from build123d import *

# Parameters (mm, degrees)
BOSS_EXTRUDE1_DEPTH = 20
SKETCH3_R           = 1
CUT_EXTRUDE1_DEPTH  = 10
SKETCH4_R           = 1
CUT_EXTRUDE2_DEPTH  = 10


with BuildPart() as part:
    # Sketch1 → Boss-Extrude1 (new body)
    with BuildSketch(Plane.XY):
        Polygon((0, 0), (58, 0), (58, 60), (61, 60), (61, -3), (-3, -3), (-3, 60), (0, 60), align=None)
    extrude(amount=-BOSS_EXTRUDE1_DEPTH)

    # Sketch3 → Cut-Extrude1 (cut)
    with BuildSketch(Plane(origin=(61, 0, 0), x_dir=(0, 0, -1), z_dir=(1, 0, 0))):
        with Locations((10, 57.541077174)):
            Circle(SKETCH3_R)
        with Locations((10, 30.375)):
            Circle(SKETCH3_R)
        Polygon((10, 32.55), (16, 32.55), (16, 55.366077174), (10, 55.366077174), (4, 55.366077174), (4, 32.55), align=None)
    extrude(amount=-CUT_EXTRUDE1_DEPTH, mode=Mode.SUBTRACT)

    # Sketch4 → Cut-Extrude2 (cut)
    with BuildSketch(Plane(origin=(0, 0, 0), x_dir=(1, 0, 0), z_dir=(0, 1, 0))):
        with Locations((19, 10)):
            Circle(SKETCH4_R)
        with Locations((39, 10)):
            Circle(SKETCH4_R)
    extrude(amount=-CUT_EXTRUDE2_DEPTH, mode=Mode.SUBTRACT)


solid = part.part
Check sheet for the modelled part. Datum: model origin and axes. Units: mm. A direction names the side the tool comes from. Give positions to 0.01 mm unless a question says otherwise; leave off trailing zeros. Order: outer loops, then holes, each group sorted by start corner. A loop starts at its lowest first (then second) coordinate and runs counter-clockwise, first axis right, second up. Notation, with made-up numbers: (-24, 47) - (27, 47) arc R11 ccw to (27, 66) - close; hole circle Ø9 at (-30.75, 23). An arc over 180 degrees is marked (long way). Answer as CSV lines item,"result".
1. Go/stop test with flat-tipped pins: P1, Ø3, axis at y = 57.54, z = -10, coming from the +X side; P2, Ø2.5, axis at x = 19, z = -10, coming from the +Y side. Record where each tip stops, or that it passes through.
Result sheet:
P1,"x = 61"
P2,"y = 0"
2. Section check D-D (y = 42.5). Record the boundary of the cut face in (x, z), then the cut area to 3 significant figures.
Result sheet:
outline,"(-3, -20) - (0, -20) - (0, 0) - (-3, 0) - close; (58, -20) - (61, -20) - (61, -16) - (58, -16) - close; (58, -4) - (61, -4) - (61, 0) - (58, 0) - close"
area,"84.0 mm²"
3. Mould release check, pull along Y, two halves, no side actions. Record for faces 1 (the face through (59, 60, -10)), 2 (the face through (60, 32.55, -10)), 3 (the face through (18.263, -1.479, -10.676)), 4 (the face through (60, 44, -16)): released by +Y, released by -Y, zero draft, split by the parting line, or undercut.
Result sheet:
face 1,"released by +Y"
face 2,"undercut"
face 3,"zero draft"
face 4,"undercut"
4. Tool access check on faces 5 (the face through (59.521, 31.366, -9.87)), 6 (the face through (29, -2, 0)), 7 (the face through (29, 0, -10)). Record the directions out of +Z, -Z, +X, -X, +Y, -Y that give a thin tool (end or side, any length) a straight path to the whole face; none if there is none.
Result sheet:
face 5,"+X"
face 6,"+Z, +X, -X, +Y, -Y"
face 7,"+Z, -Z, +Y"
5. Section check A-A (x = 19). Record the boundary of the cut face in (y, z).
Result sheet:
outline,"(-3, -20) - (0, -20) - (0, -11) - (-3, -11) - close; (-3, -9) - (0, -9) - (0, 0) - (-3, 0) - close"
6. Scan lines: probe 1 along X at (y, z) = (-1.4, -10); probe 2 along Y at (x, z) = (60.2, -10) (3 decimals); probe 3 along X at (y, z) = (17.5, -10.75). Record each from-to range of solid material in increasing order. Write a range as from..to.
Result sheet:
probe 1,"-3..18, 20..38, 40..61"
probe 2,"-3..29.375, 31.375..32.55, 55.366..56.541, 58.541..60"
probe 3,"-3..0, 58..61"
7. Section check C-C (y = 17.5). Record the boundary of the cut face in (x, z), then the cut area to 3 significant figures.
Result sheet:
outline,"(-3, -20) - (0, -20) - (0, 0) - (-3, 0) - close; (58, -20) - (61, -20) - (61, 0) - (58, 0) - close"
area,"120 mm²"
8. Section check B-B (z = -10). Record the boundary of the cut face in (x, y) (3 decimals), then the cut area to 3 significant figures.
Result sheet:
outline,"(-3, -3) - (18, -3) - (18, 0) - (0, 0) - (0, 60) - (-3, 60) - close; (20, -3) - (38, -3) - (38, 0) - (20, 0) - close; (40, -3) - (61, -3) - (61, 29.375) - (58, 29.375) - (58, 0) - (40, 0) - close; (58, 31.375) - (61, 31.375) - (61, 32.55) - (58, 32.55) - close; (58, 55.366) - (61, 55.366) - (61, 56.541) - (58, 56.541) - close; (58, 58.541) - (61, 58.541) - (61, 60) - (58, 60) - close"
area,"460 mm²"
